from build123d import *

# Parameters (mm, degrees)
SKETCH1_W           = 45.55
SKETCH1_H           = 123.67
SKETCH1_R           = 1.75
BOSS_EXTRUDE1_DEPTH = 1.65
SKETCH2_W           = 45.55
SKETCH2_H           = 123.67
BOSS_EXTRUDE2_DEPTH = 2.85
SKETCH3_W           = 8.75
SKETCH3_H           = 89.25
BOSS_EXTRUDE3_DEPTH = 11
SKETCH4_W           = 1.5
SKETCH4_H           = 83.5
CUT_EXTRUDE1_DEPTH  = 7


with BuildPart() as part:
    # Sketch1 → Boss-Extrude1 (new body)
    with BuildSketch(Plane(origin=(0, 0, 0), x_dir=(1, 0, 0), z_dir=(0, 1, 0))):
        Rectangle(SKETCH1_W, SKETCH1_H)
        with Locations((-19.154293565, -37.379539044)):
            Circle(SKETCH1_R, mode=Mode.SUBTRACT)
        with Locations((-19.154293565, 57.171070526)):
            Circle(SKETCH1_R, mode=Mode.SUBTRACT)
        with Locations((19.154293565, -37.379539044)):
            Circle(SKETCH1_R, mode=Mode.SUBTRACT)
        with Locations((19.154293565, 57.171070526)):
            Circle(SKETCH1_R, mode=Mode.SUBTRACT)
    extrude(amount=BOSS_EXTRUDE1_DEPTH)

    # Sketch2 → Boss-Extrude2 (add)
    with BuildSketch(Plane.XZ):
        Rectangle(SKETCH2_W, SKETCH2_H)
    extrude(amount=BOSS_EXTRUDE2_DEPTH)

    # Sketch3 → Boss-Extrude3 (add)
    with BuildSketch(Plane(origin=(0, 1.65, 0), x_dir=(1, 0, 0), z_dir=(0, 1, 0))):
        with Locations((6.9, 17.21)):
            Rectangle(SKETCH3_W, SKETCH3_H)
    extrude(amount=BOSS_EXTRUDE3_DEPTH)

    # Sketch4 → Cut-Extrude1 (cut)
    with BuildSketch(Plane(origin=(0, 12.65, 0), x_dir=(1, 0, 0), z_dir=(0, 1, 0))):
        with Locations((6.9, 18.085)):
            Rectangle(SKETCH4_W, SKETCH4_H)
    extrude(amount=-CUT_EXTRUDE1_DEPTH, mode=Mode.SUBTRACT)


solid = part.part
Geometry check sheet. Reference: the model listing, model coordinates, mm. A direction names the side the tool comes from. Give positions to 0.01 mm unless a question says otherwise; leave off trailing zeros. Order: outer loops, then holes, each group sorted by start corner. A loop starts at its lowest first (then second) coordinate and runs counter-clockwise, first axis right, second up.
1. Depth check by flat-ended pin: pin 1 (4.5 mm diameter, centred on x = 19.15, z = 37.38, fed in from +Y); pin 2 (4.5 mm diameter, centred on x = 6.5, y = 5, fed in from +Z) (3 decimals); pin 3 (3.5 mm diameter, centred on y = 10.5, z = -24, fed in from -X) (3 decimals). Enter the tip coordinate at first touch or a pass-through.
Completed:
pin 1: stops at y = 1.65
pin 2: stops at z = 27.415
pin 3: stops at x = 2.525
2. Access from +Z, -Z, +X, -X, +Y, -Y to the whole of each face (thin tool, end or side, straight path). Record for faces 1 (the face through (-20.4, 0.8, -58.4)), 2 (the face through (7, 7, 27.415)), 3 (the face through (22.775, -1, -1)), 4 (the face through (11.275, 7, -17)), 5 (the face through (-22.775, -1, -1)).
Completed:
face 1: +Y
face 2: +Z, +X, -X, +Y
face 3: +Z, -Z, +X, +Y, -Y
face 4: +Z, -Z, +X, +Y
face 5: +Z, -Z, -X, +Y, -Y
3. Draft check along Z on faces 6 (the face through (2.525, 7, -17)), 7 (the face through (6.15, 9, -18)), 8 (the face through (0, -1, 61.835)). Enter one of: pulls with the +Z half, pulls with the -Z half, needs draft (parallel to the pull), parting line crosses it, or undercut.
Completed:
face 6: needs draft
face 7: undercut
face 8: pulls with the +Z half
4. Sectioned sample at C-C (x = -18.5). Record the boundary of the cut face in (y, z) (3 decimals), then the cut area to 3 significant figures.
Completed:
outline: (-2.85, -61.835) - (1.65, -61.835) - (1.65, -58.794) - (0, -58.794) - (0, -55.548) - (1.65, -55.548) - (1.65, 35.756) - (0, 35.756) - (0, 39.003) - (1.65, 39.003) - (1.65, 61.835) - (-2.85, 61.835) - close
area: 546 mm2
5. Scan lines: line 1 (X direction, y = 7.5, z = -28.5) (3 decimals); line 2 (Z direction, x = 3.5, y = 4.75) (3 decimals); line 3 (Y direction, x = -8, z = -54.5). Record each from-to range of solid material in increasing order.
Completed:
line 1: x = 2.525 to 6.15, 7.65 to 11.275
line 2: z = -61.835 to 27.415
line 3: y = -2.85 to 1.65
6. Sectioned sample at A-A (z = -26). Record the boundary of the cut face in (x, y) (3 decimals), then the cut area to 3 significant figures.
Completed:
outline: (-22.775, -2.85) - (22.775, -2.85) - (22.775, 1.65) - (11.275, 1.65) - (11.275, 12.65) - (7.65, 12.65) - (7.65, 5.65) - (6.15, 5.65) - (6.15, 12.65) - (2.525, 12.65) - (2.525, 1.65) - (-22.775, 1.65) - close
area: 291 mm2
7. Sectioned sample at D-D (x = -0.5). Record the boundary of the cut face in (y, z) (3 decimals).
Completed:
outline: (-2.85, -61.835) - (1.65, -61.835) - (1.65, 61.835) - (-2.85, 61.835) - close
8. Sectioned sample at B-B (y = 6.75). Record the boundary of the cut face in (x, z) (3 decimals), then the cut area to 3 significant figures.
Completed:
outline: (2.525, -61.835) - (11.275, -61.835) - (11.275, 27.415) - (2.525, 27.415) - close; hole (6.15, -59.835) - (7.65, -59.835) - (7.65, 23.665) - (6.15, 23.665) - close
area: 656 mm2
